Source: CAD feature listing. Evaluate the final solid. Frame: model axes, mm. A direction names the side the tool comes from. Round coordinates to 2 decimals unless told otherwise and drop trailing zeros. Loops run counter-clockwise (first coordinate to the right, second up) from the corner with the lowest first, then second, coordinate; pieces in that order, holes last.
Item 1: Section query D-D on z = 6.5. Return loops of the section in (x, y).
Item 2: Section query C-C on z = 0. Return loops of the section in (x, y) (3 decimals).
Item 3: Pull-direction query (Z, two-part tool) for faces 3 (the cylindrical face through (16.86, 9.93, -5.31)), 4 (the flat face through (0, 3, -21.435)), 5 (the flat face through (-11, 15, -11)); classes: released by +Z, released by -Z, zero draft, split by the parting line, or undercut.
Item 4: Ray query, L1, parallel to X at y = 12.25, z = 0 (3 decimals); L2, parallel to Z at x = 10, y = 0.5 (3 decimals); L3, parallel to Z at x = 13, y = 1.5 (1 decimal). Return the intervals inside material, ascending.
Item 5: Section query A-A on x = 0. Return loops of the section in (y, z) (3 decimals), then the cut area to 3 significant figures.
Item 6: Section query B-B on y = 2.25. Return loops of the section in (x, z) (3 decimals).
Item 7: Access query for faces 1 (the flat face through (-15, 3, 20)), 2 (the flat face through (30, 2, 0)). Directions: +Z, -Z, +X, -X, +Y, -Y. A direction counts if a zero-diameter tool reaches every point of the face in a straight line with its end or side. Return the directions, or none.
Item 8: First-contact query: P1, Ø4.5, axis at y = 10, z = 0, coming from the -X side (3 decimals); P2, Ø1.7, axis at y = 10, z = 0, coming from the +X side; P3, Ø6, axis at y = 10, z = 7, coming from the +X side; P4, Ø4, axis at x = 2, y = 11, coming from the -Z side (3 decimals). Flat tips, straight axial feed; report the tip coordinate or a pass-through.
```python
from build123d import *

# Parameters (mm, degrees)
CROQUIS1_W                 = 60
CROQUIS1_H                 = 48
SALIENTE_EXTRUIR1_DEPTH    = 5
CROQUIS2_R                 = 17.675
SALIENTE_EXTRUIR2_DEPTH    = 10
CORTAR_EXTRUIR1_REACH      = 17
CROQUIS3_R                 = 14.675
CROQUIS5_W                 = 30
CROQUIS5_H                 = 2.87
CORTAR_EXTRUIR2_DEPTH      = 6
CROQUIS6_R                 = 1.435
CORTAR_EXTRUIR3_DEPTH      = 31
CORTAR_EXTRUIR3_DEPTH_BACK = 31


with BuildPart() as part:
    # Croquis1 → Saliente-Extruir1 (new body)
    with BuildSketch(Plane(origin=(0, 0, 0), x_dir=(1, 0, 0), z_dir=(0, 1, 0))):
        Rectangle(CROQUIS1_W, CROQUIS1_H)
    extrude(amount=SALIENTE_EXTRUIR1_DEPTH)

    # Croquis2 → Saliente-Extruir2 (add)
    with BuildSketch(Plane(origin=(0, 5, 0), x_dir=(1, 0, 0), z_dir=(0, 1, 0))):
        Circle(CROQUIS2_R)
    extrude(amount=SALIENTE_EXTRUIR2_DEPTH)

    # Croquis3 → Cortar-Extruir1 (cut, up to next)
    with BuildSketch(Plane.XZ, mode=Mode.PRIVATE) as cortar_extruir1_sk1:
        Circle(CROQUIS3_R)
    cortar_extruir1_tool1 = extrude(cortar_extruir1_sk1.sketch, amount=-CORTAR_EXTRUIR1_REACH, mode=Mode.PRIVATE) & part.part
    add(cortar_extruir1_tool1.solids().sort_by_distance((0, 0, 0))[0], mode=Mode.SUBTRACT)

    # Croquis5 → Cortar-Extruir2 (cut, through all)
    with BuildSketch(Plane(origin=(0, 5, 0), x_dir=(1, 0, 0), z_dir=(0, 1, 0))):
        with Locations((0, 20)):
            Rectangle(CROQUIS5_W, CROQUIS5_H)
        with Locations((0, -20)):
            Rectangle(CROQUIS5_W, CROQUIS5_H)
    extrude(amount=-CORTAR_EXTRUIR2_DEPTH, mode=Mode.SUBTRACT)

    # Croquis6 → Cortar-Extruir3 (cut, two sides)
    with BuildSketch(Plane(origin=(0, 0, 0), x_dir=(0, 0, -1), z_dir=(1, 0, 0))) as cortar_extruir3_sk:
        with Locations((0, 10)):
            Circle(CROQUIS6_R)
    extrude(amount=CORTAR_EXTRUIR3_DEPTH, mode=Mode.SUBTRACT)
    extrude(cortar_extruir3_sk.sketch, amount=-CORTAR_EXTRUIR3_DEPTH_BACK, mode=Mode.SUBTRACT)


solid = part.part
```
Data:
1. outline: (-30, 0) - (-13.16, 0) - (-13.16, 15) - (-16.44, 15) - (-16.44, 5) - (-30, 5) - close; (13.16, 0) - (30, 0) - (30, 5) - (16.44, 5) - (16.44, 15) - (13.16, 15) - close
2. outline: (-30, 0) - (-14.675, 0) - (-14.675, 8.565) - (-17.675, 8.565) - (-17.675, 5) - (-30, 5) - close; (-17.675, 11.435) - (-14.675, 11.435) - (-14.675, 15) - (-17.675, 15) - close; (14.675, 0) - (30, 0) - (30, 5) - (17.675, 5) - (17.675, 8.565) - (14.675, 8.565) - close; (14.675, 11.435) - (17.675, 11.435) - (17.675, 15) - (14.675, 15) - close
3. face 3: split by the parting line
3. face 4: undercut
3. face 5: zero draft
4. L1: x = -17.675 to -14.675, 14.675 to 17.675
4. L2: z = -24 to -21.435, -18.565 to -10.74, 10.74 to 18.565, 21.435 to 24
4. L3: z = -24 to -21.4, -18.6 to -6.8, 6.8 to 18.6, 21.4 to 24
5. outline: (0, -24) - (5, -24) - (5, -21.435) - (0, -21.435) - close; (0, -18.565) - (5, -18.565) - (5, -17.675) - (15, -17.675) - (15, -14.675) - (0, -14.675) - close; (0, 14.675) - (15, 14.675) - (15, 17.675) - (5, 17.675) - (5, 18.565) - (0, 18.565) - close; (0, 21.435) - (5, 21.435) - (5, 24) - (0, 24) - close
5. area: 125 mm2
6. outline: (-30, -24) - (30, -24) - (30, 24) - (-30, 24) - close; hole (-15, -21.435) - (15, -21.435) - (15, -18.565) - (-15, -18.565) - close; hole (-15, 18.565) - (15, 18.565) - (15, 21.435) - (-15, 21.435) - close; hole circle Ø29.35 at (0, 0)
7. face 1: +Y, -Y
7. face 2: +Z, -Z, +X, +Y, -Y
8. P1: stops at x = -17.675
8. P2: passes through
8. P3: stops at x = 17.22
8. P4: stops at z = -17.675
